Here's how the part is built. I have some questions about the finished solid (model axes, mm). Coordinates: 2 decimals unless noted, no trailing zeros. Write each loop counter-clockwise with the first axis right and the second up, starting at its lowest first coordinate (ties: lowest second). Pieces come first, ordered by that corner, then holes.
Autodesk Inventor part; units mm, degrees
ref_plane "YZ Plane" through (0, 0, 0) normal (1, 0, 0) x (0, 1, 0)
ref_plane "XZ Plane" through (0, 0, 0) normal (0, 1, 0) x (-1, 0, 0)
ref_plane "XY Plane" through (0, 0, 0) normal (0, 0, 1) x (1, 0, 0)
sketch "Sketch1" plane through (0, 0, 0) normal (0, 1, 0) x (-1, 0, 0)
  line L0 (0, 0) -> (-101.981, 0)
  line L1 (-101.981, 0) -> (-101.981, -86.614)
  line L2 (-101.981, -86.614) -> (0, -86.614)
  line L3 (0, -86.614) -> (0, 0)
  circle A0 centre (-8.5085, -8.5085) radius 3.4925
  circle A1 centre (-78.1055, -8.5085) radius 3.4925
  circle A2 centre (-8.5085, -78.1055) radius 3.4925
  circle A3 centre (-78.1055, -78.1055) radius 3.4925
  circle A4 centre (-43.3338, -43.3338) radius 38.1
  circle A5 centre (-94.2975, -19.05) radius 3.5
  circle A6 centre (-94.2975, -69.85) radius 3.5
  dimension "d0" = 101.981
  dimension "d1" = 86.614
  dimension "d2" = 6.985
  dimension "d3" = 8.5085
  dimension "d4" = 8.5085
  dimension "d7" = 69.597
  dimension "d10" = 69.597
  dimension "d13" = 76.2
  dimension "d14" = 43.3338
  dimension "d15" = 43.3338
  dimension "d16" = 7
  dimension "d19" = 50.8
  dimension "d24" = 19.05
  dimension "d27" = 7.6835
extrude "Extrusion1" add sketch "Sketch1" along normal blind 3.175
properties part number "MotorPlate"
1) We'd pull the mould along X, two halves only. Please class faces 1 (the face through (97.794, 1.565, -19.204)), 2 (the face through (0, 2, -44)), 3 (the face through (52, 2, -86.614)), 4 (the face through (101.981, 2, -43)): pulls with the +X half, pulls with the -X half, needs draft (parallel to the pull), parting line crosses it, or undercut.
Values follow:
face 1: undercut
face 2: pulls with the -X half
face 3: needs draft
face 4: pulls with the +X half
2) Imagine slicing it at C-C on z = -27. Please give me the cut outline in (x, y) (3 decimals), then the cut area to 3 significant figures.
Values follow:
outline: (0, 0) - (8.913, 0) - (8.913, 3.175) - (0, 3.175) - close; (77.755, 0) - (101.981, 0) - (101.981, 3.175) - (77.755, 3.175) - close
area: 105 mm2
3) Imagine slicing it at D-D on x = 92. Please give me the cut outline in (y, z) (3 decimals), then the cut area to 3 significant figures.
Values follow:
outline: (0, -86.614) - (3.175, -86.614) - (3.175, -72.49) - (0, -72.49) - close; (0, -67.21) - (3.175, -67.21) - (3.175, -21.69) - (0, -21.69) - close; (0, -16.41) - (3.175, -16.41) - (3.175, 0) - (0, 0) - close
area: 241 mm2
4) I need wall thicknesses on probe 1 along Z at (x, y) = (43.5, 0.5); probe 2 along X at (y, z) = (1.95, -11); probe 3 along X at (y, z) = (2.1, -8.5). Which ranges of each line are inside material? Lowest first, please.
Values follow:
probe 1: z = -86.61 to -81.43, -5.23 to 0
probe 2: x = 0 to 6.06, 10.96 to 23.18, 63.49 to 75.66, 80.55 to 101.98
probe 3: x = 0 to 5.02, 12 to 27.9, 58.77 to 74.61, 81.6 to 101.98
5) Will this pin go through, and if not, where does the flat tip stop? pin 1 (5.5 mm diameter, centred on x = 78.11, z = -78.11, fed in from +Y).
Values follow:
pin 1: passes through
6) Imagine slicing it at B-B on z = -17.5. Please give me the cut outline in (x, y) (3 decimals).
Values follow:
outline: (0, 0) - (15.33, 0) - (15.33, 3.175) - (0, 3.175) - close; (71.338, 0) - (91.159, 0) - (91.159, 3.175) - (71.338, 3.175) - close; (97.436, 0) - (101.981, 0) - (101.981, 3.175) - (97.436, 3.175) - close
7) Imagine slicing it at A-A on x = 46. Please give me the cut outline in (y, z) (3 decimals).
Values follow:
outline: (0, -86.614) - (3.175, -86.614) - (3.175, -81.34) - (0, -81.34) - close; (0, -5.327) - (3.175, -5.327) - (3.175, 0) - (0, 0) - close
